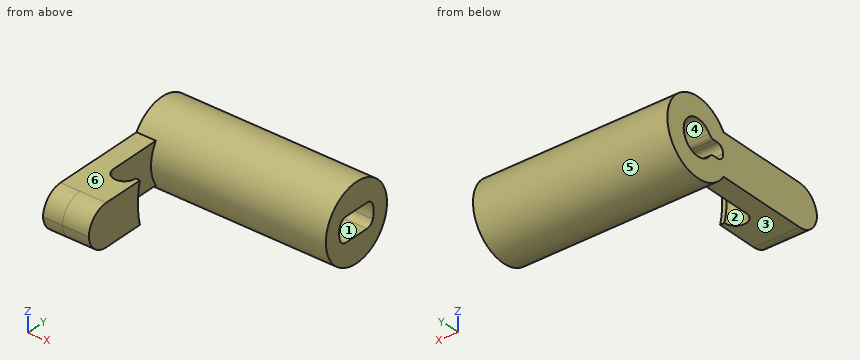
from build123d import *

# Parameters (mm, degrees)
SKETCH1_R           = 8.7376
BOSS_EXTRUDE1_DEPTH = 45.085
BOSS_EXTRUDE3_DEPTH = 4.516000112
FILLET2_R           = 5
BOSS_EXTRUDE4_DEPTH = 6.096
CUT_EXTRUDE8_DEPTH  = 6.096
CUT_EXTRUDE10_DEPTH = 12.192
FILLET11_R          = 1.778
SKETCH25_R          = 2.5527
CUT_EXTRUDE14_DEPTH = 59.077319733
CUT_EXTRUDE15_DEPTH = 9.525
FILLET12_R          = 1.5875


with BuildPart() as part:
    # Sketch1 → Boss-Extrude1 (new body)
    with BuildSketch(Plane.YZ):
        with Locations(Location((0, 0, 0), (0, 0, 270))):
            Circle(SKETCH1_R)
    extrude(amount=BOSS_EXTRUDE1_DEPTH)

    # Sketch10 → Boss-Extrude3 (add)
    with BuildSketch(Plane(origin=(0, 0, 0), x_dir=(0, -1, 0), z_dir=(-1, 0, 0))):
        with BuildLine():
            Line((7.325588544, 4.7625), (34.036, 4.7625))
            Line((34.036, 4.7625), (34.036, -4.7625))
            Line((34.036, -4.7625), (7.325588544, -4.7625))
            ThreePointArc((7.325588544, -4.7625), (8.7376, 0), (7.325588544, 4.7625))
        make_face()
    extrude(amount=-BOSS_EXTRUDE3_DEPTH)

    # Fillet2
    # the kernel refuses this fillet: 5 mm, written as the material it takes off along each edge
    with BuildSketch(Plane(origin=(-12.5, -34.036, 4.7625), x_dir=(0, 1, 0), z_dir=(1, 0, 0))) as fillet2_piece_1:
        with BuildLine():
            CenterArc((FILLET2_R, -FILLET2_R), FILLET2_R, 90, 90)
            Line((0, -FILLET2_R), (0, 0))
            Line((0, 0), (FILLET2_R, 0))
        make_face()
    extrude(amount=29.516000112, mode=Mode.SUBTRACT)
    with BuildSketch(Plane(origin=(-12.5, -34.036, -4.7625), x_dir=(0, 1, 0), z_dir=(1, 0, 0))) as fillet2_piece_2:
        with BuildLine():
            CenterArc((FILLET2_R, FILLET2_R), FILLET2_R, 180, 90)
            Line((0, FILLET2_R), (0, 0))
            Line((0, 0), (FILLET2_R, 0))
        make_face()
    extrude(amount=29.516000112, mode=Mode.SUBTRACT)

    # Sketch15 → Boss-Extrude4 (add)
    with BuildSketch(Plane.YZ.offset(4.516000112)):
        with BuildLine():
            Line((-18.79035619, -4.7625), (-18.79035619, 4.7625))
            Line((-18.79035619, 4.7625), (-29.036, 4.7625))
            ThreePointArc((-29.036, 4.7625), (-32.486543435, 3.381028707), (-34.03035619, 0))
            ThreePointArc((-34.03035619, 0), (-32.486543435, -3.381028707), (-29.036, -4.7625))
            Line((-29.036, -4.7625), (-18.79035619, -4.7625))
        make_face()
    extrude(amount=BOSS_EXTRUDE4_DEPTH)

    # Sketch21 → Cut-Extrude8 (cut)
    with BuildSketch(Plane.YZ.offset(10.612000112)):
        with BuildLine():
            Line((-19.42535619, -4.7625), (-18.79035619, -4.7625))
            Line((-18.79035619, -4.7625), (-18.79035619, 4.7625))
            Line((-18.79035619, 4.7625), (-19.42535619, 4.7625))
            ThreePointArc((-19.42535619, 4.7625), (-19.991344097, 0), (-19.42535619, -4.7625))
        make_face()
    extrude(amount=-CUT_EXTRUDE8_DEPTH, mode=Mode.SUBTRACT)

    # Sketch22 → Cut-Extrude10 (cut)
    with BuildSketch(Plane.YZ.offset(45.085)):
        with BuildLine():
            Line((-4.089715516, -2.794), (4.089715516, -2.794))
            ThreePointArc((4.089715516, -2.794), (4.953, 0), (4.089715516, 2.794))
            Line((4.089715516, 2.794), (-4.089715516, 2.794))
            ThreePointArc((-4.089715516, 2.794), (-4.953, 0), (-4.089715516, -2.794))
        make_face()
    extrude(amount=-CUT_EXTRUDE10_DEPTH, mode=Mode.SUBTRACT)

    # Fillet11
    fillet11_edges = [part.edges().sort_by_distance(p)[0] for p in [
        (38.989, 4.089715516, 2.794),
        (38.989, 4.089715516, -2.794),
        (38.989, -4.089715516, -2.794),
        (38.989, -4.089715516, 2.794),
    ]]
    fillet(fillet11_edges, radius=FILLET11_R)

    # Sketch25 → Cut-Extrude14 (cut, through all)
    with BuildSketch(Plane(origin=(0, 0, -4.7625), x_dir=(1, 0, 0), z_dir=(0, 0, -1))):
        with Locations((7.068700112, 19.42535619)):
            Circle(SKETCH25_R)
    extrude(amount=-CUT_EXTRUDE14_DEPTH, mode=Mode.SUBTRACT)

    # Sketch26 → Cut-Extrude15 (cut)
    with BuildSketch(Plane(origin=(0, 0, 0), x_dir=(0, -1, 0), z_dir=(-1, 0, 0))):
        with BuildLine():
            Line((3.684641875, 1.7145), (7.177141875, 1.7145))
            Line((7.177141875, 1.7145), (7.177141875, -1.7145))
            Line((7.177141875, -1.7145), (3.684641875, -1.7145))
            ThreePointArc((3.684641875, -1.7145), (-4.064, 0), (3.684641875, 1.7145))
        make_face()
    extrude(amount=-CUT_EXTRUDE15_DEPTH, mode=Mode.SUBTRACT)

    # Fillet12
    fillet12_edges = [part.edges().sort_by_distance(p)[0] for p in [
        (4.7625, -3.684641875, -1.7145),
        (4.7625, -3.684641875, 1.7145),
        (4.7625, -7.177141875, 1.7145),
        (4.7625, -7.177141875, -1.7145),
    ]]
    fillet(fillet12_edges, radius=FILLET12_R)


solid = part.part
Source: CAD feature listing. Evaluate the final solid. Frame: model axes, mm. Face numbers are marked on the shaded views. A direction names the side the tool comes from. Round coordinates to 2 decimals unless told otherwise and drop trailing zeros. Loops run counter-clockwise (first coordinate to the right, second up) from the corner with the lowest first, then second, coordinate; pieces in that order, holes last.
Q1. Section B-B, the plane z = 3.5. Return loops of the section in (x, y) (3 decimals).
Q2. First-contact query: P1, Ø8, axis at y = -28.5, z = -6, coming from the +X side; P2, Ø8.5, axis at x = 6, y = -14, coming from the +Z side; P3, Ø11.5, axis at x = 7, y = -22, coming from the -Z side. Flat tips, straight axial feed; report the tip coordinate or a pass-through.
Q3. Section C-C, the plane x = 18. Return loops of the section in (y, z), plus the area to 3 significant figures.
Q4. Ray query, line 1 (Y direction, x = 6.5, z = 0); line 2 (Z direction, x = 4, y = 0); line 3 (X direction, y = -13.5, z = -2.75). Return the intervals inside material, ascending.
Q5. Mould query, pull axis Z, two halves, no side actions, for the marked faces 4, 5 and 6. Classes: pulls with the +Z half, pulls with the -Z half, needs draft (parallel to the pull), parting line crosses it, or undercut.
Q6. Access query for the marked faces 1, 2 and 3. Directions: +Z, -Z, +X, -X, +Y, -Y. A direction counts if a zero-diameter tool reaches every point of the face in a straight line with its end or side. Return the directions, or none.
Q7. Section A-A, the plane y = 0. Return loops of the section in (x, z) (3 decimals).
Q8. Section D-D, the plane y = -22.5. Return loops of the section in (x, z), plus the area to 3 significant figures.
Solutions:
1. outline: (0, -32.357) - (10.612, -32.357) - (10.612, -19.688) - (9.608, -19.688) arc R2.553 cw to (4.53, -19.688) - (4.516, -19.688) - (4.516, -8.006) - (45.085, -8.006) - (45.085, 8.006) - (0, 8.006) - (0, 2.065) - (9.525, 2.065) - (9.525, -2.065) - (0, -2.065) - close
2. P1: stops at x = 10.61
2. P2: stops at z = 4.76
2. P3: stops at z = -4.76
3. outline: circle Ø17.48 at (0, 0)
3. area: 240 mm2
4. line 1: y = -34.03 to -21.91, -8.74 to -7.18, 4.06 to 8.74
4. line 2: z = -8.74 to -4.06, 4.06 to 8.74
4. line 3: x = 0 to 4.52
5. face 4: undercut
5. face 5: parting line crosses it
5. face 6: pulls with the +Z half
6. face 1: +X
6. face 2: +Z, -Z
6. face 3: -Z, +X, -X, -Y
7. outline: (0, -8.738) - (45.085, -8.738) - (45.085, -2.794) - (32.893, -2.794) - (32.893, 2.794) - (45.085, 2.794) - (45.085, 8.738) - (0, 8.738) - (0, 4.064) - (9.525, 4.064) - (9.525, -4.064) - (0, -4.064) - close
8. outline: (0, -4.76) - (10.61, -4.76) - (10.61, 4.76) - (0, 4.76) - close
8. area: 101 mm2
